from build123d import *

# Parameters (mm, degrees)
RESSALTO_EXTRUS_O1_DEPTH      = 2
RESSALTO_EXTRUS_O1_DEPTH_BACK = 1
ESBO_O1_3_W                   = 35
ESBO_O1_3_H                   = 2
RESSALTO_EXTRUS_O2_DEPTH      = 8
RESSALTO_EXTRUS_O3_DEPTH      = 8
RESSALTO_EXTRUS_O5_START      = 8
ESBO_O1_5_W                   = 3
ESBO_O1_5_H                   = 50
ESBO_O1_5_W_2                 = 22
ESBO_O1_5_H_2                 = 6
RESSALTO_EXTRUS_O5_DEPTH      = 6.2
RESSALTO_EXTRUS_O6_START      = 14
ESBO_O1_6_W                   = 2
ESBO_O1_6_H                   = 6
ESBO_O1_6_H_2                 = 2
ESBO_O1_6_W_2                 = 22
ESBO_O1_6_W_3                 = 6
ESBO_O1_6_W_4                 = 3
ESBO_O1_6_H_3                 = 38
RESSALTO_EXTRUS_O6_DEPTH      = 5
ESBO_O5_R                     = 1.5
CORTE_EXTRUS_O2_DEPTH         = 10
RESSALTO_EXTRUS_O7_START      = -2
ESBO_O6_W                     = 13
ESBO_O6_H                     = 19
ESBO_O6_R                     = 1.5
ESBO_O6_W_2                   = 14
ESBO_O6_H_2                   = 7
RESSALTO_EXTRUS_O7_DEPTH      = 2
RESSALTO_EXTRUS_O8_START      = -10
ESBO_O6_3_W                   = 45
ESBO_O6_3_H                   = 0.8
RESSALTO_EXTRUS_O8_DEPTH      = 8
ESBO_O7_W                     = 2
ESBO_O7_H                     = 3.59531288
CORTE_EXTRUS_O3_DEPTH         = 10
ESBO_O11_W                    = 80
ESBO_O11_H                    = 3
RESSALTO_EXTRUS_O11_DEPTH     = 20
ESBO_O12_W                    = 3
ESBO_O12_H                    = 25
RESSALTO_EXTRUS_O12_DEPTH     = 18
RESSALTO_EXTRUS_O9_START      = -3
RESSALTO_EXTRUS_O9_DEPTH      = 3
ESBO_O10_W                    = 10
ESBO_O10_H                    = 25
RESSALTO_EXTRUS_O10_DEPTH     = 3
ESBO_O13_W                    = 4.849706681
ESBO_O13_H                    = 25
CORTE_EXTRUS_O4_DEPTH         = 10
RESSALTO_EXTRUS_O13_REACH     = 84.522
ESBO_O14_W                    = 1
ESBO_O14_H                    = 20.8
ESBO_O15_W                    = 1
ESBO_O15_H                    = 20
RESSALTO_EXTRUS_O14_DEPTH     = 39
ESBO_O20_W                    = 8
ESBO_O20_H                    = 10
RESSALTO_EXTRUS_O18_DEPTH     = 10
CORTE_EXTRUS_O6_START         = -10
ESBO_O21_R                    = 1.5
CORTE_EXTRUS_O6_DEPTH         = 10
RESSALTO_EXTRUS_O19_DEPTH     = 1
CORTE_EXTRUS_O7_DEPTH         = 4
RESSALTO_EXTRUS_O20_DEPTH     = 10
FILETE1_R                     = 1


with BuildPart() as part:
    # Esboço1 → Ressalto-extrusão1 (new, two sides: drawn at the far end of the back side and taken through both)
    with BuildSketch(Plane(origin=(0, 0, 0), x_dir=(1, 0, 0), z_dir=(0, 1, 0)).offset(-RESSALTO_EXTRUS_O1_DEPTH_BACK)):
        Polygon((0, 0), (0, 50), (20, 50), (20, 10), (35, 10), (35, 0), align=None)
    extrude(amount=RESSALTO_EXTRUS_O1_DEPTH + RESSALTO_EXTRUS_O1_DEPTH_BACK)

    # Esboço1<3> → Ressalto-extrusão2 (add)
    with BuildSketch(Plane(origin=(0, 0, 0), x_dir=(1, 0, 0), z_dir=(0, 1, 0))):
        with Locations((17.5, 1)):
            Rectangle(ESBO_O1_3_W, ESBO_O1_3_H)
        with Locations((17.5, 9)):
            Rectangle(ESBO_O1_3_W, ESBO_O1_3_H)
    extrude(amount=RESSALTO_EXTRUS_O2_DEPTH)

    # Esboço1<4> → Ressalto-extrusão3 (add)
    with BuildSketch(Plane(origin=(0, 0, 0), x_dir=(1, 0, 0), z_dir=(0, 1, 0))):
        Polygon((0, 10), (3, 10), (3, 48), (9, 48), (9, 10), (11, 10), (11, 50), (0, 50), align=None)
    extrude(amount=RESSALTO_EXTRUS_O3_DEPTH)

    # Esboço1<5> → Ressalto-extrusão5 (add)
    # profile 1 of 2: a face of its own
    with BuildSketch(Plane(origin=(0, 0, 0), x_dir=(1, 0, 0), z_dir=(0, 1, 0)).offset(RESSALTO_EXTRUS_O5_START)):
        with Locations((1.5, 25)):
            Rectangle(ESBO_O1_5_W, ESBO_O1_5_H)
    # profile 2 of 2: a face of its own
    with BuildSketch(Plane(origin=(0, 0, 0), x_dir=(1, 0, 0), z_dir=(0, 1, 0)).offset(RESSALTO_EXTRUS_O5_START)):
        Polygon((35, 0), (35, 10), (11, 10), (11, 50), (9, 50), (9, 0), align=None)
        with Locations((22, 5)):
            Rectangle(ESBO_O1_5_W_2, ESBO_O1_5_H_2, mode=Mode.SUBTRACT)
    extrude(amount=RESSALTO_EXTRUS_O5_DEPTH)

    # Esboço1<6> → Ressalto-extrusão6 (add)
    with BuildSketch(Plane(origin=(0, 0, 0), x_dir=(1, 0, 0), z_dir=(0, 1, 0)).offset(RESSALTO_EXTRUS_O6_START)):
        with Locations((34, 5)):
            Rectangle(ESBO_O1_6_W, ESBO_O1_6_H)
        with Locations((34, 1)):
            Rectangle(ESBO_O1_6_W, ESBO_O1_6_H_2)
        with Locations((22, 1)):
            Rectangle(ESBO_O1_6_W_2, ESBO_O1_6_H_2)
        with Locations((34, 9)):
            Rectangle(ESBO_O1_6_W, ESBO_O1_6_H_2)
        Polygon((11, 10), (11, 8), (33, 8), (33, 10), (20, 10), align=None)
        with Locations((10, 1)):
            Rectangle(ESBO_O1_6_W, ESBO_O1_6_H_2)
        with Locations((6, 1)):
            Rectangle(ESBO_O1_6_W_3, ESBO_O1_6_H_2)
        with Locations((1.5, 1)):
            Rectangle(ESBO_O1_6_W_4, ESBO_O1_6_H_2)
        with Locations((1.5, 5)):
            Rectangle(ESBO_O1_6_W_4, ESBO_O1_6_H)
        with Locations((1.5, 9)):
            Rectangle(ESBO_O1_6_W_4, ESBO_O1_6_H_2)
        with Locations((1.5, 29)):
            Rectangle(ESBO_O1_6_W_4, ESBO_O1_6_H_3)
        with Locations((1.5, 49)):
            Rectangle(ESBO_O1_6_W_4, ESBO_O1_6_H_2)
        with Locations((6, 9)):
            Rectangle(ESBO_O1_6_W_3, ESBO_O1_6_H_2)
        with Locations((10, 9)):
            Rectangle(ESBO_O1_6_W, ESBO_O1_6_H_2)
        with Locations((6, 49)):
            Rectangle(ESBO_O1_6_W_3, ESBO_O1_6_H_2)
        with Locations((10, 49)):
            Rectangle(ESBO_O1_6_W, ESBO_O1_6_H_2)
        with Locations((10, 29)):
            Rectangle(ESBO_O1_6_W, ESBO_O1_6_H_3)
    extrude(amount=RESSALTO_EXTRUS_O6_DEPTH)

    # Esboço5 → Corte-extrusão2 (cut)
    with BuildSketch(Plane(origin=(0, 2, 0), x_dir=(1, 0, 0), z_dir=(0, 1, 0))):
        with Locations(Location((16, 15, 0), (0, 0, 270))):
            Circle(ESBO_O5_R)
        with Locations(Location((16, 45, 0), (0, 0, 270))):
            Circle(ESBO_O5_R)
    extrude(amount=-CORTE_EXTRUS_O2_DEPTH, mode=Mode.SUBTRACT)

    # Esboço6 → Ressalto-extrusão7 (add)
    with BuildSketch(Plane.XY.offset(RESSALTO_EXTRUS_O7_START)):
        Polygon((80, 44.8), (0, 44.8), (0, 19), (35, 19), (35, -1), (80, -1), align=None)
        with Locations((14.5, 33.3)):
            Rectangle(ESBO_O6_W, ESBO_O6_H, mode=Mode.SUBTRACT)
        with Locations((34, 32.731591612)):
            Circle(ESBO_O6_R, mode=Mode.SUBTRACT)
        Polygon((45, 23.231591612), (40, 28.231591612), (40, 42.231591612), (67.2, 42.231591612), (67.2, 28.231591612), (62.2, 23.231591612), align=None, mode=Mode.SUBTRACT)
        with Locations((73.2, 32.731591612)):
            Circle(ESBO_O6_R, mode=Mode.SUBTRACT)
        with Locations((54, 13.5)):
            Rectangle(ESBO_O6_W_2, ESBO_O6_H_2, mode=Mode.SUBTRACT)
    extrude(amount=RESSALTO_EXTRUS_O7_DEPTH)

    # Esboço6<3> → Ressalto-extrusão8 (add)
    with BuildSketch(Plane.XY.offset(RESSALTO_EXTRUS_O8_START)):
        Polygon((80, 19.8), (0, 19.8), (0, 19), (35, 19), (80, 19), align=None)
        with Locations((57.5, 18.6)):
            Rectangle(ESBO_O6_3_W, ESBO_O6_3_H)
    extrude(amount=RESSALTO_EXTRUS_O8_DEPTH)

    # Esboço7 → Corte-extrusão3 (cut)
    with BuildSketch(Plane(origin=(0, 19.8, 0), x_dir=(1, 0, 0), z_dir=(0, 1, 0))):
        with Locations((44, 5.971535205)):
            Rectangle(ESBO_O7_W, ESBO_O7_H)
        with Locations((64, 5.971535205)):
            Rectangle(ESBO_O7_W, ESBO_O7_H)
    extrude(amount=-CORTE_EXTRUS_O3_DEPTH, mode=Mode.SUBTRACT)

    # Esboço11 → Ressalto-extrusão11 (add)
    with BuildSketch(Plane.XY):
        with Locations((40, 46.3)):
            Rectangle(ESBO_O11_W, ESBO_O11_H)
    extrude(amount=-RESSALTO_EXTRUS_O11_DEPTH)

    # Esboço12 → Ressalto-extrusão12 (add)
    with BuildSketch(Plane(origin=(0, 0, -2), x_dir=(-1, 0, 0), z_dir=(0, 0, -1))):
        with Locations((-26.5, 32.3)):
            Rectangle(ESBO_O12_W, ESBO_O12_H)
    extrude(amount=RESSALTO_EXTRUS_O12_DEPTH)

    # Esboço9 → Ressalto-extrusão9 (add)
    with BuildSketch(Plane.ZY.offset(RESSALTO_EXTRUS_O9_START)):
        Polygon((-20, 47.8), (-50, 19), (-2, 19), (-2, 47.8), align=None)
    extrude(amount=RESSALTO_EXTRUS_O9_DEPTH)

    # Esboço10 → Ressalto-extrusão10 (add)
    with BuildSketch(Plane(origin=(80, 0, 0), x_dir=(0, 0, -1), z_dir=(1, 0, 0))):
        with Locations((5, 32.3)):
            Rectangle(ESBO_O10_W, ESBO_O10_H)
    extrude(amount=-RESSALTO_EXTRUS_O10_DEPTH)

    # Esboço13 → Corte-extrusão4 (cut)
    with BuildSketch(Plane(origin=(28, 0, 0), x_dir=(0, 0, -1), z_dir=(1, 0, 0))):
        with Locations((22.424853341, 32.3)):
            Rectangle(ESBO_O13_W, ESBO_O13_H)
        Polygon((10, 19.8), (20, 44.8), (20, 19.8), align=None)
    extrude(amount=-CORTE_EXTRUS_O4_DEPTH, mode=Mode.SUBTRACT)

    # Ressalto-extrusão13: up to this face of the body (flat: up to its plane)
    ressalto_extrus_o13_end = Plane(part.part.faces().sort_by_distance((11, 10.5, -30))[0])
    # Esboço14 → Ressalto-extrusão13 (add, up to the picked face)
    with BuildSketch(Plane(origin=(35, 0, 0), x_dir=(0, 0, -1), z_dir=(1, 0, 0)), mode=Mode.PRIVATE) as ressalto_extrus_o13_sk1:
        with Locations((10.5, 9.4)):
            Rectangle(ESBO_O14_W, ESBO_O14_H)
    ressalto_extrus_o13_tool1 = split(extrude(ressalto_extrus_o13_sk1.sketch, amount=-RESSALTO_EXTRUS_O13_REACH, mode=Mode.PRIVATE), bisect_by=ressalto_extrus_o13_end, keep=Keep.BOTH, mode=Mode.PRIVATE)
    add(ressalto_extrus_o13_tool1.solids().sort_by(Axis((35, 9.4, -10.5), (-1, 0, 0)))[0])

    # Esboço15 → Ressalto-extrusão14 (add)
    with BuildSketch(Plane(origin=(0, 0, -50), x_dir=(-1, 0, 0), z_dir=(0, 0, -1))):
        with Locations((-11.5, 9)):
            Rectangle(ESBO_O15_W, ESBO_O15_H)
    extrude(amount=-RESSALTO_EXTRUS_O14_DEPTH)

    # Esboço20 → Ressalto-extrusão18 (add)
    with BuildSketch(Plane(origin=(0, 2, 0), x_dir=(1, 0, 0), z_dir=(0, 1, 0))):
        with Locations((16, 16)):
            Rectangle(ESBO_O20_W, ESBO_O20_H)
    extrude(amount=RESSALTO_EXTRUS_O18_DEPTH)

    # Esboço21 → Corte-extrusão6 (cut)
    with BuildSketch(Plane.XZ.offset(-2).offset(CORTE_EXTRUS_O6_START)):
        with Locations(Location((16, -15, 0), (0, 0, 270))):
            Circle(ESBO_O21_R)
    extrude(amount=CORTE_EXTRUS_O6_DEPTH, mode=Mode.SUBTRACT)

    # Esboço22 → Ressalto-extrusão19 (add)
    with BuildSketch(Plane(origin=(0, 0, -10), x_dir=(-1, 0, 0), z_dir=(0, 0, -1))):
        Polygon((-35, 18.2), (-35, 19.8), (-77, 19.8), (-77, 44.8), (-80, 44.8), (-80, 18.2), align=None)
    extrude(amount=RESSALTO_EXTRUS_O19_DEPTH)

    # Esboço23 → Corte-extrusão7 (cut)
    with BuildSketch(Plane(origin=(0, 12, 0), x_dir=(1, 0, 0), z_dir=(0, 1, 0))):
        Polygon((18.75, 16.58771324), (16, 18.175426481), (13.25, 16.58771324), (13.25, 13.41228676), (16, 11.824573519), (18.75, 13.41228676), align=None)
        Polygon((18.75, 43.41228676), (18.75, 46.58771324), (16, 48.175426481), (13.25, 46.58771324), (13.25, 43.41228676), (16, 41.824573519), align=None)
    extrude(amount=-CORTE_EXTRUS_O7_DEPTH, mode=Mode.SUBTRACT)

    # Esboço24 → Ressalto-extrusão20 (add)
    with BuildSketch(Plane(origin=(80, 0, 0), x_dir=(0, 0, -1), z_dir=(1, 0, 0))):
        with BuildLine():
            Line((9.100514075, 8.213270058), (2, 18.2))
            Line((2, 18.2), (2, 5.55))
            ThreePointArc((2, 5.55), (3.951321001, 7.864048246), (6.935535628, 7.357159696))
            Line((6.935535628, 7.357159696), (6.984313483, 7.25))
            Line((6.984313483, 7.25), (9.100514075, 8.213270058))
        make_face()
        with BuildLine():
            Line((2, 4.45), (2, -1))
            Line((2, -1), (9.100514075, -1))
            Line((9.100514075, -1), (9.100514075, 1.559444743))
            Line((9.100514075, 1.559444743), (6.984313483, 2.75))
            Line((6.984313483, 2.75), (6.320880397, 2.25085923))
            ThreePointArc((6.320880397, 2.25085923), (3.616556582, 2.281804954), (2, 4.45))
        make_face()
    extrude(amount=-RESSALTO_EXTRUS_O20_DEPTH)

    # Filete1
    # the kernel refuses this fillet: 1 mm, written as the material it takes off along each edge
    with BuildSketch(Plane(origin=(81.633402331, 2.75, -6.984313483), x_dir=(0, -0.4903214392898115, -0.8715416720804391), z_dir=(-1, 0, 0))) as filete1_piece_1:
        with BuildLine():
            CenterArc((FILETE1_R * 0.653360932246, FILETE1_R), FILETE1_R, 203.681935757, 66.318064243)
            Line((-FILETE1_R * 0.262428341882, FILETE1_R * 0.598340933885), (-FILETE1_R * 0.280744127364, FILETE1_R * 0.590307752563))
            Line((-FILETE1_R * 0.280744127364, FILETE1_R * 0.590307752563), (-FILETE1_R * 0.0130672186449, -FILETE1_R * 0.02))
            Line((-FILETE1_R * 0.0130672186449, -FILETE1_R * 0.02), (FILETE1_R * 0.653360932246, -FILETE1_R * 0.02))
            Line((FILETE1_R * 0.653360932246, -FILETE1_R * 0.02), (FILETE1_R * 0.653360932246, 0))
        make_face()
    extrude(amount=13.266804661, mode=Mode.SUBTRACT)
    with BuildSketch(Plane(origin=(81.176901612, 7.25, -6.984313483), x_dir=(0, 0.910145890185138, 0.4142878933532846), z_dir=(-1, 0, 0))) as filete1_piece_2:
        with BuildLine():
            CenterArc((1, 0.470760645), FILETE1_R, 180, 28.083682979)
            Line((0, 0.470760645), (-0.02, 0.470760645))
            Line((-0.02, 0.470760645), (-0.02, 0))
            Line((-0.02, 0), (0, -0.02))
            ThreePointArc((0, -0.02), (0.058869516, -0.02), (0.100093813, -0.009415213))
            Line((0.100093813, -0.009415213), (0.117739032, 0))
        make_face()
    extrude(amount=12.353803225, mode=Mode.SUBTRACT)


solid = part.part
The listing builds one solid part. Answer for the finished solid, in the listing's coordinates (mm). A direction names the side the tool comes from. Coordinates: 2 decimals unless noted, no trailing zeros. Write each loop counter-clockwise with the first axis right and the second up, starting at its lowest first coordinate (ties: lowest second). Pieces come first, ordered by that corner, then holes. Notation, with made-up numbers: (-2, 27.5) - (18, 27.5) arc R29 cw to (18, 53.5) - close; hole circle Ø8 at (49.5, -21). An arc over 180 degrees is marked (long way). Put each result on its own line as item: value.
1. Find the intervals of material crossed by line 1 along X through (y, z) = (39, -7); line 2 along X through (y, z) = (11, -5); line 3 along Z through (x, y) = (16, 4.55), in increasing order. Write a range as from..to.
Answer sheet:
line 1: x = 0..3, 25..28, 77..80
line 2: x = 0..3, 9..11, 33..35, 70..80
line 3: z = -21..-16.5, -13.5..-8, -2..0
2. The part is cut by section D-D on z = -33. Give the vertices of the cut face in (x, y).
Answer sheet:
outline: (0, -1) - (20, -1) - (20, 2) - (12, 2) - (12, 19) - (9, 19) - (9, 2) - (3, 2) - (3, 35.32) - (0, 35.32) - close
3. A tool of negligible diameter and unlimited length cuts with its end or side. For faces 1 (the face through (16, 7, -21)), 2 (the face through (15.9, 12, -18.3)), 3 (the face through (17.36, 10.03, -12.61)), 4 (the face through (54, 17, -1)), from which of +Z, -Z, +X, -X, +Y, -Y can it reach the whole face along a straight path? Write none if from no direction.
Answer sheet:
face 1: -Z, +X, +Y
face 2: -Z, +X
face 3: none
face 4: +Z, -Z
4. The part is cut by section C-C on y = 26. Give the vertices of the cut face in (x, z).
Answer sheet:
outline: (0, -42.71) - (3, -42.71) - (3, -2) - (8, -2) - (8, 0) - (0, 0) - close; (21, -2) - (25, -2) - (25, -12.48) - (28, -12.48) - (28, -2) - (42.23, -2) - (42.23, 0) - (21, 0) - close; (64.97, -2) - (77, -2) - (77, -11) - (80, -11) - (80, 0) - (64.97, 0) - close
5. Flat-ended cylindrical pins translate along their axes: pin 1 Ø5 at (x, z) = (16, -15) entering from -Y; pin 2 Ø0.9 at (x, y) = (29.5, 46.5) entering from -Z; pin 3 Ø5.5 at (x, z) = (46, -15) entering from -Y; pin 4 Ø3 at (x, y) = (40, 12) entering from -Z. Find the tip coordinate at first contact, or state that the pin passes through.
Answer sheet:
pin 1: stops at y = -1
pin 2: stops at z = -20
pin 3: stops at y = 44.8
pin 4: stops at z = -2
6. The part is cut by section B-B on x = 34. Give the vertices of the cut face in (y, z), plus the area to 3 significant figures.
Answer sheet:
outline: (-1, -11) - (19.8, -11) - (19.8, -2) - (31.23, -2) - (31.23, 0) - (-1, 0) - close; (34.23, -2) - (44.8, -2) - (44.8, -20) - (47.8, -20) - (47.8, 0) - (34.23, 0) - close; hole (2, -8) - (8, -8) - (8, -2) - (2, -2) - close
area: 297 mm^2
7. Determine the mould class of faces 5 (the face through (33, 14, -11)), 6 (the face through (13.25, 10, -15)), 7 (the face through (80, 29, -5)) for opening direction X: pulls with the +X half, pulls with the -X half, needs draft (parallel to the pull), parting line crosses it, or undercut.
Answer sheet:
face 5: needs draft
face 6: undercut
face 7: pulls with the +X half
8. The part is cut by section A-A on z = -15. Give the vertices of the cut face in (x, y), plus the area to 3 significant figures.
Answer sheet:
outline: (0, -1) - (14.5, -1) - (14.5, 8) - (13.25, 8) - (13.25, 12) - (12, 12) - (12, 19) - (9, 19) - (9, 2) - (3, 2) - (3, 44.8) - (25, 44.8) - (25, 32.3) - (28, 32.3) - (28, 44.8) - (80, 44.8) - (80, 47.8) - (0, 47.8) - close; (17.5, -1) - (20, -1) - (20, 12) - (18.75, 12) - (18.75, 8) - (17.5, 8) - close
area: 548 mm^2
